```python
from build123d import *

# Parameters (mm, degrees)
F0_W        = 5.9436
F0_H        = 6.223
F1_DEPTH    = 3.5
F2_R        = 1.75
F3_DEPTH    = 2.5
F3_TAPER    = 1.5
F4_R        = 0.1
F5_R        = 0.5
F6_DEPTH    = 0.5
F7_R        = 0.49999
F8_W        = 0.7
F8_H        = 0.3
F11_SIZE2   = 0.5
F11_SIZE    = 0.2
F11_2_SIZE2 = 0.5
F11_2_SIZE  = 0.2


# Not quite as in the source:
# - a fillet or chamfer is up to 0.001 mm smaller than in the source, because OpenCascade refuses the exact size


with BuildPart() as f1:
    # F0 (on Top) → F1 (new body)
    with BuildSketch(Plane.XY):
        Rectangle(F0_W, F0_H)
    extrude(amount=F1_DEPTH)

    # F2 (on face) → F3 (join)
    with BuildSketch(Plane.XY.offset(3.5)):
        Circle(F2_R)
    extrude(amount=F3_DEPTH, taper=F3_TAPER)

    # F4
    f4_edges = [f1.edges().sort_by_distance(p)[0] for p in [
        (2.9718, -3.1115, 1.75),
        (-2.9718, -3.1115, 1.75),
        (-2.9718, 3.1115, 1.75),
        (2.9718, 3.1115, 1.75),
        (2.9718, 0, 3.5),
        (0, -3.1115, 3.5),
        (-2.9718, 0, 3.5),
        (0, 3.1115, 3.5),
    ]]
    fillet(f4_edges, radius=F4_R)

    # F5 (on face) → F6 (join)
    with BuildSketch(Plane.XY.offset(3.5)):
        with Locations((2.3, -2.3)):
            Circle(F5_R)
        with Locations((2.3, 2.3)):
            Circle(F5_R)
        with Locations((-2.3, 2.3)):
            Circle(F5_R)
        with Locations((-2.3, -2.3)):
            Circle(F5_R)
    extrude(amount=F6_DEPTH)

    # F7 (radius 0.5 in the source; OpenCascade refuses exactly that, so slightly less here)
    f7_edges = [f1.edges().sort_by_distance(p)[0] for p in [
        (1.8, -2.3, 4),
        (1.8, 2.3, 4),
        (-2.8, 2.3, 4),
        (-2.8, -2.3, 4),
    ]]
    fillet(f7_edges, radius=F7_R)

    # F10: sweep along a path in F9
    with BuildLine(Plane.YZ) as f10_path:
        Line((-3.1115, 1.15), (-3.1615, 1.15))
        ThreePointArc((-3.1615, 1.15), (-3.2675660172, 1.1060660172), (-3.3115, 1))
        Line((-3.3115, 1), (-3.3115, -3.35))
    # F8 (on face) → F10 (sweep)
    with BuildSketch(Plane.XZ.offset(3.1115)):
        with Locations((-2.25, 1.15)):
            Rectangle(F8_W, F8_H)
        with Locations((2.25, 1.15)):
            Rectangle(F8_W, F8_H)
    sweep(path=f10_path.line)

    # F11
    f11_edges = [f1.edges().sort_by_distance(p)[0] for p in [
        (-2.6, -3.3115, -3.35),
        (-1.9, -3.3115, -3.35),
    ]]
    f11_side = f1.faces().sort_by_distance((-2.25, -3.3115, -3.35))[0]
    chamfer(f11_edges, length=F11_SIZE, length2=F11_SIZE2, reference=f11_side)

    # F11#2
    f11_2_edges = [f1.edges().sort_by_distance(p)[0] for p in [
        (1.9, -3.3115, -3.35),
        (2.6, -3.3115, -3.35),
    ]]
    f11_2_side = f1.faces().sort_by_distance((2.25, -3.3115, -3.35))[0]
    chamfer(f11_2_edges, length=F11_2_SIZE, length2=F11_2_SIZE2, reference=f11_2_side)

    # F12: F1 across plane


with BuildPart() as f1_1:
    add(f1.part)
    add(f1.part.mirror(Plane.XZ))


solid = f1_1.part
```
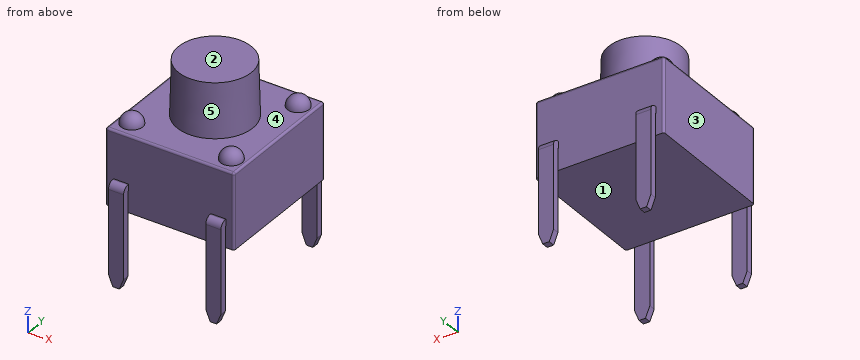
Design review of the part built by this model. Coordinates are the model's own, in mm. Face numbers are marked on the shaded views. A direction names the side the tool comes from. Coordinates: 2 decimals unless noted, no trailing zeros. Loops run counter-clockwise (first coordinate to the right, second up) from the corner with the lowest first, then second, coordinate; pieces in that order, holes last. Notation, with made-up numbers: (-13, 75) - (3, 75) arc R20 ccw to (3, 81) - close; hole circle Ø9 at (7, 69.5). An arc over 180 degrees is marked (long way). Use CSV: the item, a comma, the result in double quotes. Start each with the question number.
1) For pin 1 Ø1.7 at (x, z) = (0.5, 2) entering from +Y; pin 2 Ø1.5 at (x, z) = (0.5, 0.5) entering from -Y, all flat-tipped, find the tip position at first contact; note any pin that passes through.
2) Wall thickness on L1, parallel to Y at x = -2.35, z = -1.5; L2, parallel to Z at x = -1.2, y = -1; L3, parallel to Z at x = 0.35, y = 2.5: over which ranges is each line inside the solid? List them lowest first. Write a range as from..to.
3) Consider section C-C on z = 4.25. Write out the cut boundary in (x, y).
4) Consider section D-D on z = 5.25. Write out the cut boundary in (x, y).
5) Consider section A-A on y = 0. Write out the cut boundary in (x, z).
6) Tool access review of the marked faces 1 and 2: name each direction out of +Z, -Z, +X, -X, +Y, -Y from which nothing blocks a thin tool from reaching the whole face with its end or side.
7) The part is to be moulded in two halves that separate along Y. For the marked faces 3, 4 and 5, say which applies: +Y half, -Y half, draft (parallel to the pull), parting line (faces both ways), or undercut.
8) Consider section B-B on z = 2.5. Write out the cut boundary in (x, y).
Geometry says:
1,pin 1,"y = 3.11"
1,pin 2,"y = -3.11"
2,L1,"-3.46..-3.16, 3.16..3.46"
2,L2,"0..6"
2,L3,"0..3.5"
3,outline,"circle Ø3.46 at (0, 0)"
4,outline,"circle Ø3.41 at (0, 0)"
5,outline,"(-2.97, 0) - (2.97, 0) - (2.97, 3.4) arc R0.1 ccw to (2.87, 3.5) - (1.75, 3.5) - (1.68, 6) - (-1.68, 6) - (-1.75, 3.5) - (-2.87, 3.5) arc R0.1 ccw to (-2.97, 3.4) - close"
6,face 1,"-Z, +X, -X"
6,face 2,"+Z, +X, -X, +Y, -Y"
7,face 3,"draft"
7,face 4,"undercut"
7,face 5,"parting line"
8,outline,"(-2.97, -3.01) arc R0.1 ccw to (-2.87, -3.11) - (2.87, -3.11) arc R0.1 ccw to (2.97, -3.01) - (2.97, 3.01) arc R0.1 ccw to (2.87, 3.11) - (-2.87, 3.11) arc R0.1 ccw to (-2.97, 3.01) - close"
